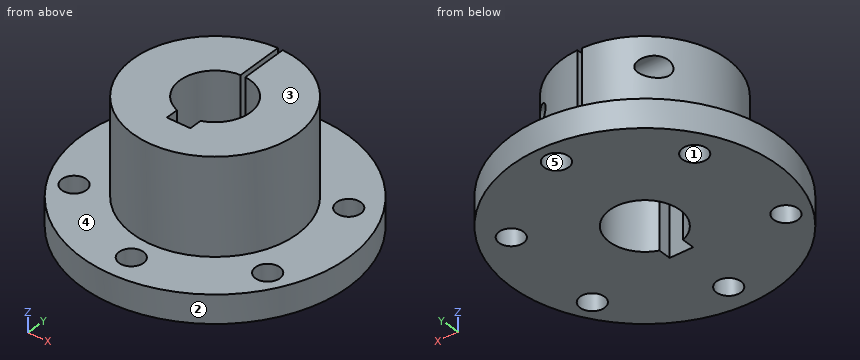
from build123d import *

# Parameters (mm, degrees)
SKETCH_2_R               = 2.6
CUT_EXTRUDE_1_DEPTH      = 49.063291606
SKETCH_3_W               = 5
SKETCH_3_H               = 3.3
CUT_EXTRUDE_2_DEPTH      = 49.063291606
CUT_EXTRUDE_START        = 12
SKETCH_4_W               = 1
SKETCH_4_H               = 11
CUT_EXTRUDE_3_DEPTH      = 14.4
CUT_EXTRUDE_4_DEPTH      = 49.063291606
CUT_EXTRUDE_4_DEPTH_BACK = 49.063291606
SKETCH_5_R               = 2.25


with BuildPart() as part:
    # 草图1 → 旋转1 (revolve)
    with BuildSketch(Plane(origin=(0, 0, 0), x_dir=(0, 0, -1), z_dir=(1, 0, 0)), mode=Mode.PRIVATE) as revolve_1_sk:
        Polygon((0, 7.5), (0, 28.4), (-6, 28.4), (-6, 17.5), (-26.4, 17.5), (-26.4, 7.5), align=None)
    revolve(revolve_1_sk.sketch.rotate(Axis((0, 0, 31.4), (0, 0, -1)), 90), axis=Axis((0, 0, 31.4), (0, 0, -1)))

    # 草图2 → 切除-拉伸1 (cut, through all)
    with BuildSketch(Plane.XY):
        with Locations(Location((0, 23.75, 0), (0, 0, 180))):
            Circle(SKETCH_2_R)
        with Locations(Location((-20.56810334, -11.875, 0), (0, 0, 180))):
            Circle(SKETCH_2_R)
        with Locations(Location((20.56810334, -11.875, 0), (0, 0, 180))):
            Circle(SKETCH_2_R)
        with Locations(Location((19.485571585, 11.25, 0), (0, 0, 180))):
            Circle(SKETCH_2_R)
        with Locations(Location((-19.485571585, 11.25, 0), (0, 0, 180))):
            Circle(SKETCH_2_R)
        with Locations(Location((0, -22.5, 0), (0, 0, 180))):
            Circle(SKETCH_2_R)
    extrude(amount=CUT_EXTRUDE_1_DEPTH, mode=Mode.SUBTRACT)

    # 草图3 → 切除-拉伸2 (cut, through all)
    with BuildSketch(Plane.XY):
        with Locations((0, -8.15)):
            Rectangle(SKETCH_3_W, SKETCH_3_H)
    extrude(amount=CUT_EXTRUDE_2_DEPTH, mode=Mode.SUBTRACT)

    # 草图4 → 切除-拉伸3 (cut)
    with BuildSketch(Plane.XY.offset(CUT_EXTRUDE_START)):
        with Locations((0, 12.5)):
            Rectangle(SKETCH_4_W, SKETCH_4_H)
    extrude(amount=CUT_EXTRUDE_3_DEPTH, mode=Mode.SUBTRACT)

    # 草图5 → 切除-拉伸4 (cut, two sides: drawn at the far end of the back side and taken through both)
    with BuildSketch(Plane(origin=(0, 0, 0), x_dir=(0, 0, -1), z_dir=(1, 0, 0)).offset(-CUT_EXTRUDE_4_DEPTH_BACK)):
        with Locations((-20.2, 12.5)):
            Circle(SKETCH_5_R)
    extrude(amount=CUT_EXTRUDE_4_DEPTH + CUT_EXTRUDE_4_DEPTH_BACK, mode=Mode.SUBTRACT)


solid = part.part
Geometry check sheet. Reference: the model listing, model coordinates, mm. Face numbers are marked on the shaded views. A direction names the side the tool comes from. Give positions to 0.01 mm unless a question says otherwise; leave off trailing zeros. Order: outer loops, then holes, each group sorted by start corner. A loop starts at its lowest first (then second) coordinate and runs counter-clockwise, first axis right, second up. Notation, with made-up numbers: (-31.75, -31) - (-18.75, -31) arc R17 cw to (-18.75, -4) - close; hole circle Ø9 at (48.25, -25.5). An arc over 180 degrees is marked (long way). Answer as a JSON object with one key per item and string values.
(1) Draft check along Y on the marked faces 1, 2 and 3. Enter one of: released by +Y, released by -Y, zero draft, split by the parting line, or undercut.
Report:
{"face 1": "undercut", "face 2": "split by the parting line", "face 3": "zero draft"}
(2) Cross-section at D-D (y = -11). Record the cut outline in (x, z).
Report:
{"outline": "(-26.18, 0) - (-23.02, 0) - (-23.02, 6) - (-26.18, 6) - close; (-18.12, 0) - (18.12, 0) - (18.12, 6) - (13.61, 6) - (13.61, 26.4) - (-13.61, 26.4) - (-13.61, 6) - (-18.12, 6) - close; (23.02, 0) - (26.18, 0) - (26.18, 6) - (23.02, 6) - close"}
(3) Tool access check on the marked faces 4 and 5. Record the directions out of +Z, -Z, +X, -X, +Y, -Y that give a thin tool (end or side, any length) a straight path to the whole face; none if there is none.
Report:
{"face 4": "+Z", "face 5": "+Z, -Z"}
(4) Material ranges on line 1 (Y direction, x = 0, z = 2.2); line 2 (X direction, y = 13.5, z = 3); line 3 (X direction, y = 11.25, z = 1.7), recorded low to high.
Report:
{"line 1": "-28.4 to -25.1, -19.9 to -9.8, 7.5 to 21.15, 26.35 to 28.4", "line 2": "-24.99 to -20.79, -18.18 to 18.18, 20.79 to 24.99", "line 3": "-26.08 to -22.09, -16.89 to 16.89, 22.09 to 26.08"}
(5) Depth check by flat-ended pin: pin 1 Ø1.4 at (y, z) = (-8.5, 12) entering from +X; pin 2 Ø1.5 at (x, y) = (19, 18.5) entering from +Z; pin 3 Ø8 at (y, z) = (11, 16.5) entering from +X; pin 4 Ø1.1 at (x, y) = (0, 13) entering from +Z. Enter the tip coordinate at first touch or a pass-through.
Report:
{"pin 1": "x = 15.67", "pin 2": "z = 6", "pin 3": "x = 16.04", "pin 4": "z = 26.4"}
(6) Cross-section at B-B (z = 10). Record the cut outline in (x, y), then the cut area to 3 significant figures.
Report:
{"outline": "circle Ø35 at (0, 0); hole (-2.5, -9.8) - (2.5, -9.8) - (2.5, -7.07) arc R7.5 ccw (long way) to (-2.5, -7.07) - close", "area": "773 mm^2"}
(7) Cross-section at C-C (y = 0). Record the cut outline in (x, z), then the cut area to 3 significant figures.
Report:
{"outline": "(-28.4, 0) - (-7.5, 0) - (-7.5, 26.4) - (-17.5, 26.4) - (-17.5, 6) - (-28.4, 6) - close; (7.5, 0) - (28.4, 0) - (28.4, 6) - (17.5, 6) - (17.5, 26.4) - (7.5, 26.4) - close", "area": "659 mm^2"}
(8) Cross-section at A-A (x = 4.5). Record the cut outline in (y, z), then the cut area to 3 significant figures.
Report:
{"outline": "(-28.04, 0) - (-6, 0) - (-6, 26.4) - (-16.91, 26.4) - (-16.91, 6) - (-28.04, 6) - close; (6, 0) - (28.04, 0) - (28.04, 6) - (16.91, 6) - (16.91, 26.4) - (6, 26.4) - close; hole circle Ø4.5 at (12.5, 20.2)", "area": "694 mm^2"}
